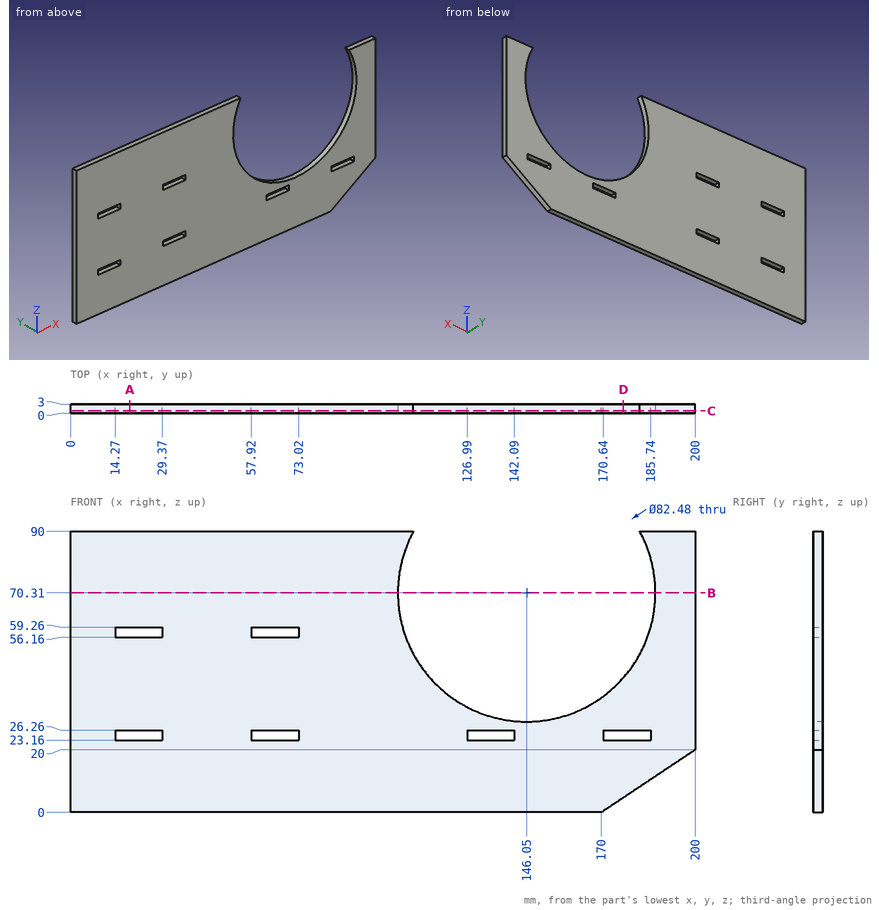
Print and shaded views of the part. All mm, measured from the part's lowest x, y and z. Round coordinates to 2 decimals unless told otherwise and drop trailing zeros. Order: outer loops, then holes, each group sorted by start corner. A loop starts at its lowest first (then second) coordinate and runs counter-clockwise, first axis right, second up.
Q1. Slice it at C-C (y = 0.8). State how many separate pieces and enclosed holes the cut face has, and give its area (3 significant figures).
Q2. Slice it at B-B (z = 70.31). Write the cut outline in (x, y).
Q3. Wall check: L1, parallel to X at y = 1.15, z = 26; L2, parallel to X at y = 1.9, z = 70.31; L3, parallel to X at y = 0.3, z = 57.5. Give the ranges that are in metal, low to high.
Q4. Drop a flat-ended pin along its axis: pin 1 (0.9 mm diameter, centred on x = 137, y = 2, fed in from +Z). Give the stop position or say it passes through.
Q5. Slice it at A-A (x = 19). Write the cut outline in (y, z), and give its area (3 significant figures).
Q6. Slice it at D-D (x = 177). Write the cut outline in (y, z) (3 decimals), and give its area (3 significant figures).
Results below:
1. separate pieces: 1
1. enclosed holes: 6
1. area: 13,200 mm2
2. outline: (0, 0) - (104.81, 0) - (104.81, 3) - (0, 3) - close; (187.29, 0) - (200, 0) - (200, 3) - (187.29, 3) - close
3. L1: x = 0 to 14.27, 29.37 to 57.92, 73.02 to 126.99, 142.09 to 170.64, 185.74 to 200
3. L2: x = 0 to 104.81, 187.29 to 200
3. L3: x = 0 to 14.27, 29.37 to 57.92, 73.02 to 106.85, 185.25 to 200
4. pin 1: stops at z = 30.18
5. outline: (0, 0) - (3, 0) - (3, 23.16) - (0, 23.16) - close; (0, 26.26) - (3, 26.26) - (3, 56.16) - (0, 56.16) - close; (0, 59.26) - (3, 59.26) - (3, 90) - (0, 90) - close
5. area: 251 mm2
6. outline: (0, 4.667) - (3, 4.667) - (3, 23.16) - (0, 23.16) - close; (0, 26.26) - (3, 26.26) - (3, 43.055) - (0, 43.055) - close
6. area: 106 mm2
